Geometry: final body of the model. Coordinates: model frame, mm. A direction names the side the tool comes from. Give positions to 0.01 mm unless a question says otherwise; leave off trailing zeros. Order: outer loops, then holes, each group sorted by start corner. A loop starts at its lowest first (then second) coordinate and runs counter-clockwise, first axis right, second up. Notation, with made-up numbers: (44.5, -37) - (98.5, -37) arc R29 ccw to (98.5, 0) - close; hole circle Ø2 at (32, 78). An arc over 180 degrees is marked (long way). One line per item, written item: value.
```python
from build123d import *

# Parameters (mm, degrees)
SKETCH1_R                    = 1
BASE_SHAPE_DEPTH             = 0.6
FILLETS_R                    = 1
M2_5_COUNTERSUNKS_AT_2_COUNT = 2
M2_5_COUNTERSUNKS_AT_2_PITCH = 73.76
M2_5_COUNTERSUNKS_AT_3_COUNT = 2
M2_5_COUNTERSUNKS_AT_3_PITCH = 73.537756289
M2_5_COUNTERSUNKS_AT_4_COUNT = 2
M2_5_COUNTERSUNKS_AT_4_PITCH = 92.959345953
M2_5_COUNTERSUNKS_AT_5_COUNT = 2
M2_5_COUNTERSUNKS_AT_5_PITCH = 36.88
M2_5_COUNTERSUNKS_AT_6_COUNT = 2
M2_5_COUNTERSUNKS_AT_6_PITCH = 72.631898864


with BuildPart() as part:
    # Sketch1 → Base shape (new body, symmetric)
    with BuildSketch(Plane(origin=(0, 0, 0), x_dir=(1, 0, 0), z_dir=(0, 1, 0))):
        with BuildLine():
            ThreePointArc((2.75, 36.88), (1.944543648, 34.935456352), (0, 34.13))
            Line((0, 34.13), (-44.1, 34.13))
            ThreePointArc((-44.1, 34.13), (-44.807106781, 33.837106781), (-45.1, 33.13))
            Line((-45.1, 33.13), (-45.1, 32.13))
            ThreePointArc((-45.1, 32.13), (-45.392893219, 31.422893219), (-46.1, 31.13))
            Line((-46.1, 31.13), (-66.992025159, 31.13))
            ThreePointArc((-66.992025159, 31.13), (-71.559934966, 29.237909806), (-73.452025159, 24.67))
            ThreePointArc((-73.452025159, 24.67), (-71.507481511, 23.864543648), (-70.702025159, 21.92))
            ThreePointArc((-70.702025159, 21.92), (-71.507481511, 19.975456352), (-73.452025159, 19.17))
            Line((-73.452025159, 19.17), (-73.452025159, 16.662625843))
            ThreePointArc((-73.452025159, 16.662625843), (-63.663567803, 10.763596053), (-59.822025159, 0))
            ThreePointArc((-59.822025159, 0), (-63.663567803, -10.763596053), (-73.452025159, -16.662625843))
            Line((-73.452025159, -16.662625843), (-73.452025159, -19.17))
            ThreePointArc((-73.452025159, -19.17), (-71.507481511, -19.975456352), (-70.702025159, -21.92))
            ThreePointArc((-70.702025159, -21.92), (-71.507481511, -23.864543648), (-73.452025159, -24.67))
            Line((-73.452025159, -24.67), (-73.452025159, -30.8))
            Line((-73.452025159, -30.8), (-63.952025159, -30.8))
            Line((-63.952025159, -30.8), (-63.952025159, -34.13))
            Line((-63.952025159, -34.13), (-63.952025159, -39.5))
            Line((-63.952025159, -39.5), (-53.952025159, -39.5))
            Line((-53.952025159, -39.5), (-53.952025159, -36.88))
            ThreePointArc((-53.952025159, -36.88), (-53.146568808, -34.935456352), (-51.202025159, -34.13))
            Line((-51.202025159, -34.13), (0, -34.13))
            ThreePointArc((0, -34.13), (1.944543648, -34.935456352), (2.75, -36.88))
            ThreePointArc((2.75, -36.88), (2.220381771, -38.502468734), (0.835523788, -39.5))
            Line((0.835523788, -39.5), (11.4, -39.5))
            Line((11.4, -39.5), (11.4, 39.5))
            Line((11.4, 39.5), (0.835523788, 39.5))
            ThreePointArc((0.835523788, 39.5), (2.220381771, 38.502468734), (2.75, 36.88))
        make_face()
        with Locations((-64.925, -21.92)):
            Circle(SKETCH1_R, mode=Mode.SUBTRACT)
        with Locations((7.075, -36.88)):
            Circle(SKETCH1_R, mode=Mode.SUBTRACT)
        with Locations((-55.497025159, 0)):
            Circle(SKETCH1_R, mode=Mode.SUBTRACT)
        with Locations((-64.925, 21.92)):
            Circle(SKETCH1_R, mode=Mode.SUBTRACT)
        with Locations((7.075, 0)):
            Circle(SKETCH1_R, mode=Mode.SUBTRACT)
        with Locations((7.075, 36.88)):
            Circle(SKETCH1_R, mode=Mode.SUBTRACT)
    extrude(amount=BASE_SHAPE_DEPTH, both=True)

    # Fillets
    fillets_edges = [part.edges().sort_by_distance(p)[0] for p in [
        (0.835523788, -0.3, -39.5),
        (11.4, -0.3, -39.5),
        (11.4, -0.3, 39.5),
        (0.835523788, -0.3, 39.5),
        (-53.952025159, -0.3, 39.5),
        (-63.952025159, -0.3, 39.5),
        (-63.952025159, -0.3, 30.8),
        (-73.452025159, -0.3, 30.8),
        (-73.452025159, -0.3, 24.67),
        (-73.452025159, -0.3, 19.17),
        (-73.452025159, -0.3, 16.662625843),
        (-73.452025159, -0.3, -16.662625843),
        (-73.452025159, -0.3, -19.17),
        (-73.452025159, -0.3, -24.67),
    ]]
    fillet(fillets_edges, radius=FILLETS_R)

    # Sketch3 → M2.5 countersunks (revolve, cut)
    with BuildSketch(Plane(origin=(7.075, -0.6, -36.88), x_dir=(0, 0, -1), z_dir=(1, 0, 0))):
        Polygon((0, 0), (0, 1.2), (1.25, 1.2), (1.25, 1.55), (2.5, 0.3), (2.5, 0), align=None)
    m2_5_countersunks = revolve(axis=Axis((7.075, -6.95, -36.88), (0, 1, 0)), mode=Mode.SUBTRACT)

    # M2.5 countersunks at 2: M2.5 countersunks ×2
    with Locations(*[(0, 0, i * M2_5_COUNTERSUNKS_AT_2_PITCH) for i in range(1, M2_5_COUNTERSUNKS_AT_2_COUNT)]):
        add(m2_5_countersunks, mode=Mode.SUBTRACT)

    # M2.5 countersunks at 3: M2.5 countersunks ×2
    with Locations(*[Vector(-0.979088888, 0, 0.203432913) * (i * M2_5_COUNTERSUNKS_AT_3_PITCH) for i in range(1, M2_5_COUNTERSUNKS_AT_3_COUNT)]):
        add(m2_5_countersunks, mode=Mode.SUBTRACT)

    # M2.5 countersunks at 4: M2.5 countersunks ×2
    with Locations(*[Vector(-0.774532128, 0, 0.632534571) * (i * M2_5_COUNTERSUNKS_AT_4_PITCH) for i in range(1, M2_5_COUNTERSUNKS_AT_4_COUNT)]):
        add(m2_5_countersunks, mode=Mode.SUBTRACT)

    # M2.5 countersunks at 5: M2.5 countersunks ×2
    with Locations(*[(0, 0, i * M2_5_COUNTERSUNKS_AT_5_PITCH) for i in range(1, M2_5_COUNTERSUNKS_AT_5_COUNT)]):
        add(m2_5_countersunks, mode=Mode.SUBTRACT)

    # M2.5 countersunks at 6: M2.5 countersunks ×2
    with Locations(*[Vector(-0.861495103, 0, 0.507765879) * (i * M2_5_COUNTERSUNKS_AT_6_PITCH) for i in range(1, M2_5_COUNTERSUNKS_AT_6_COUNT)]):
        add(m2_5_countersunks, mode=Mode.SUBTRACT)


with BuildPart() as body_2:
    # Mirror1: mirrored copy
    add(part.part.mirror(Plane.ZX))


solid = body_2.part
```
1) Section B-B, the plane x = -26.5. Return loops of the section in (y, z), then the cut area to 3 significant figures.
Answers below:
outline: (-0.6, -34.13) - (0.6, -34.13) - (0.6, 34.13) - (-0.6, 34.13) - close
area: 81.9 mm^2
2) Mould query, pull axis Z, two halves, no side actions, for faces 1 (the face through (-71.14, -0.01, -29.62)), 2 (the face through (-63.97, 0.45, 19.61)), 3 (the face through (-32, 0.6, -1)). Classes: released by +Z, released by -Z, zero draft, split by the parting line, or undercut.
Answers below:
face 1: released by -Z
face 2: undercut
face 3: zero draft
3) Set-up query: faces 4 (the face through (-70.702, -0.008, -21.945)), 5 (the face through (8.03, 0.45, -2.31)), 6 (the face through (-53.17, -0.01, 34.96)). Return all of +Z, -Z, +X, -X, +Y, -Y with unobstructed straight access to the full face (end or side cutting, diameter ignored); none if empty.
Answers below:
face 4: -X, +Y, -Y
face 5: +Y
face 6: +Z, +Y, -Y
4) Material intervals for line 1 along X through (y, z) = (-0.2, 36); line 2 along Z through (x, y) = (5.5, 0.25); line 3 along X through (y, z) = (-0.2, 0.5), sorted ascending.
Answers below:
line 1: -63.95 to -53.81, 2.61 to 5.28, 8.87 to 11.4
line 2: -39.5 to -38.76, -35 to -1.88, 1.88 to 35, 38.76 to 39.5
line 3: -59.83 to -57.43, -53.56 to 5.14, 9.01 to 11.4
5) Section A-A, the plane z = 21.92. Return loops of the section in (x, y) (3 decimals).
Answers below:
outline: (-70.702, -0.6) - (-66.525, -0.6) - (-67.425, 0.3) - (-67.425, 0.6) - (-70.702, 0.6) - close; (-63.325, -0.6) - (11.4, -0.6) - (11.4, 0.6) - (-62.425, 0.6) - (-62.425, 0.3) - close
6) Section C-C, the plane z = 0. Return loops of the section in (x, y) (3 decimals), then the cut area to 3 significant figures.
Answers below:
outline: (-59.822, -0.6) - (-57.097, -0.6) - (-57.997, 0.3) - (-57.997, 0.6) - (-59.822, 0.6) - close; (-53.897, -0.6) - (5.475, -0.6) - (4.575, 0.3) - (4.575, 0.6) - (-52.997, 0.6) - (-52.997, 0.3) - close; (8.675, -0.6) - (11.4, -0.6) - (11.4, 0.6) - (9.575, 0.6) - (9.575, 0.3) - close
area: 75.1 mm^2
7) Section D-D, the plane y = -0.35. Count the separate pieces of the cut face and the enclosed holes in it, then the cut area to 3 significant figures.
Answers below:
separate pieces: 1
enclosed holes: 6
area: 5,390 mm^2
8) First-contact query: pin 1 (4 mm diameter, centred on x = 7.075, z = 36.88, fed in from +Y); pin 2 (0.5 mm diameter, centred on y = 0, z = -32.5, fed in from -X). Flat tips, straight axial feed; report the tip coordinate or a pass-through.
Answers below:
pin 1: y = -0.2
pin 2: x = -45.1
